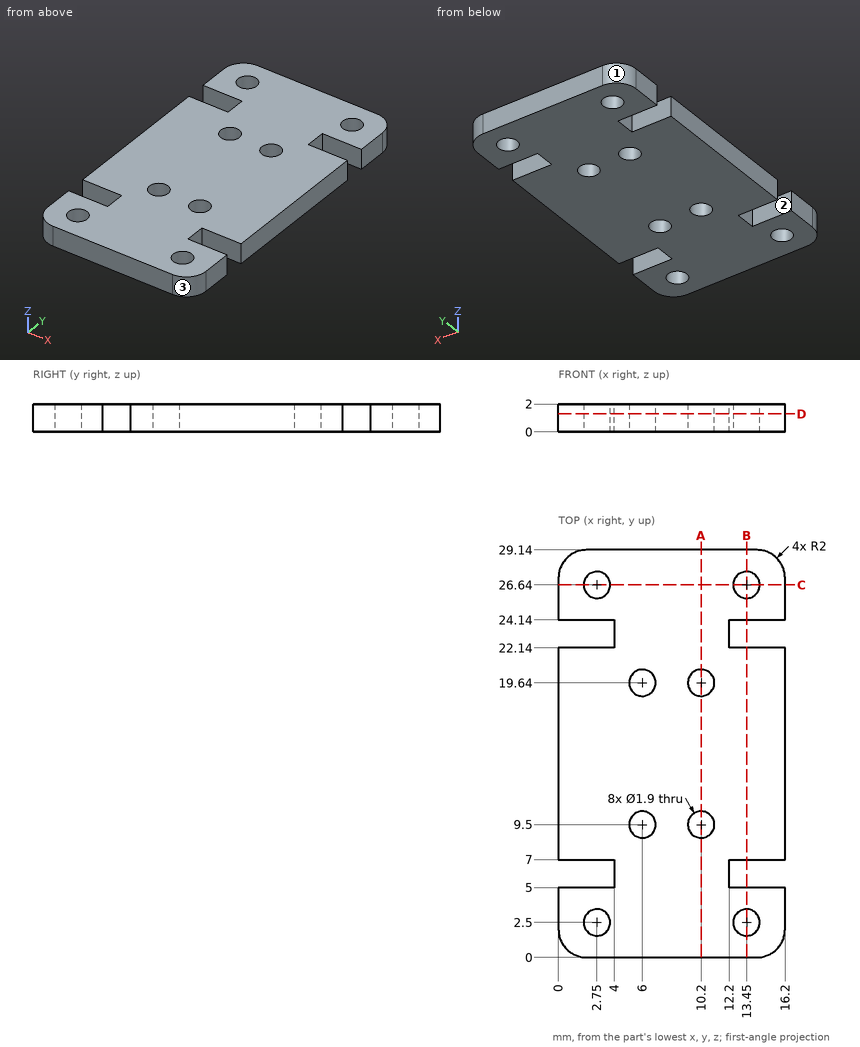
Could you check a few things on this drawing? It's one solid part, dimensions in mm from its lowest x, y, z. Round coordinates to 2 decimals unless told otherwise and drop trailing zeros. Order: outer loops, then holes, each group sorted by start corner. A loop starts at its lowest first (then second) coordinate and runs counter-clockwise, first axis right, second up. Notation, with made-up numbers: M -40,-36.5 L -11,-36.5 A19 cw -11,-12.5 Z; hole C 47.25,57.5 d6. An arc over 180 degrees is marked long. Return JSON: item names as keys, results as strings. Group by question number.
1. If we section it at B-B on x = 13.45: List the corners of the cut face in (y, z) for me.
2. If we section it at D-D on z = 1.3: State how many separate pieces and enclosed holes the cut face has, then the cut area to 3 significant figures.
3. Please list where these lines run through material, in increasing order: probe 1 along Y at (x, z) = (13.45, 1.1); probe 2 along Y at (x, z) = (10.2, 0.4); probe 3 along X at (y, z) = (19.5, 0.35).
4. If we section it at C-C on y = 26.64: List the corners of the cut face in (x, z) for me.
5. If we section it at A-A on x = 10.2: List the corners of the cut face in (y, z) for me.
6. I'm going to push flat-ended pins straight in: pin 1 Ø1 at (y, z) = (5, 0) entering from -X; pin 2 Ø0.6 at (y, z) = (6, 1) entering from +X. Where does each tip first touch, or does it pass through?
7. If we mould it in two halves opening along Y, with no side actions, what happens to the marked faces 1, 2 and 3? For each: pulls with the +Y half, pulls with the -Y half, needs draft (parallel to the pull), parting line crosses it, or undercut.
Reply:
{
 "1": {"outline": "M 0,0 L 1.55,0 L 1.55,2 L 0,2 Z; M 3.45,0 L 5,0 L 5,2 L 3.45,2 Z; M 7,0 L 22.14,0 L 22.14,2 L 7,2 Z; M 24.14,0 L 25.69,0 L 25.69,2 L 24.14,2 Z; M 27.59,0 L 29.14,0 L 29.14,2 L 27.59,2 Z"},
 "2": {"separate pieces": "1", "enclosed holes": "8", "area": "414 mm^2"},
 "3": {"probe 1": "0 to 1.55, 3.45 to 5, 7 to 22.14, 24.14 to 25.69, 27.59 to 29.14", "probe 2": "0 to 8.55, 10.45 to 18.69, 20.59 to 29.14", "probe 3": "0 to 5.06, 6.94 to 9.26, 11.14 to 16.2"},
 "4": {"outline": "M 0,0 L 1.8,0 L 1.8,2 L 0,2 Z; M 3.7,0 L 12.5,0 L 12.5,2 L 3.7,2 Z; M 14.4,0 L 16.2,0 L 16.2,2 L 14.4,2 Z"},
 "5": {"outline": "M 0,0 L 8.55,0 L 8.55,2 L 0,2 Z; M 10.45,0 L 18.69,0 L 18.69,2 L 10.45,2 Z; M 20.59,0 L 29.14,0 L 29.14,2 L 20.59,2 Z"},
 "6": {"pin 1": "x = 0", "pin 2": "x = 12.2"},
 "7": {"face 1": "pulls with the +Y half", "face 2": "undercut", "face 3": "pulls with the -Y half"}
}
